from build123d import *

# Parameters (mm, degrees)
EXTRUDE_1931_DEPTH = 2


with BuildPart() as part:
    # Sketch 231 → Revolve 1 (revolve)
    with BuildSketch(Plane.XY, mode=Mode.PRIVATE) as revolve_1_sk:
        with BuildLine():
            Line((0, 11), (0, 0))
            Line((0, 0), (1, 0))
            Line((1, 0), (1, 5.25))
            Line((1, 5.25), (3.5, 5.25))
            Line((3.5, 5.25), (3.5, 0))
            Line((3.5, 0), (11.2, 0))
            Line((11.2, 0), (11.2, 4.8))
            ThreePointArc((11.2, 4.8), (10.2627417, 7.0627417), (8, 8))
            ThreePointArc((8, 8), (7.121320344, 10.121320344), (5, 11))
            Line((5, 11), (0, 11))
        make_face()
    revolve(revolve_1_sk.sketch.rotate(Axis((0, 0, 0), (1, 0, 0)), 90), axis=Axis((0, 0, 0), (1, 0, 0)))

    # Sketch 913 → Extrude 1931 (add, symmetric)
    with BuildSketch(Plane.XY):
        with BuildLine():
            ThreePointArc((11.2, 4.4), (29.338267199, 10.995701086), (45.2, 0))
            Line((45.2, 0), (11.2, 0))
            Line((11.2, 0), (11.2, 4.4))
        make_face()
        with BuildLine():
            Line((31.263463773, 0), (11.2, 0))
            Line((11.2, 0), (11.2, -3.914978255))
            ThreePointArc((11.2, -3.914978255), (22.080678837, -6.30816882), (31.263463773, 0))
        make_face()
        Polygon((38.912013935, 0), (35.248695767, 0), (35.248695767, -11.07), (38.912013935, -4.32), align=None)
        Polygon((35.248695767, 0), (31.263463773, 0), (32.498964702, -1.197255299), (32.498964702, -9.797255299), (35.248695767, -11.07), align=None)
        Polygon((42.083014277, -1.2), (42.083014277, 0), (40.307542508, 0), (40.307542508, -6.49), align=None)
        Polygon((40.307542508, 0), (38.912013935, 0), (38.912013935, -4.32), (40.307542508, -6.49), align=None)
        Polygon((42.083014277, -1.2), (45.2, 0), (42.083014277, 0), align=None)
    extrude(amount=EXTRUDE_1931_DEPTH, both=True)


solid = part.part
Build history of the part. All positions in model axes, mm. A direction names the side the tool comes from. Give positions to 0.01 mm unless a question says otherwise; leave off trailing zeros. Order: outer loops, then holes, each group sorted by start corner. A loop starts at its lowest first (then second) coordinate and runs counter-clockwise, first axis right, second up. Notation, with made-up numbers: M 83.25,51.25 L 90.25,51.25 A9 cw 90.25,65.25 Z; hole C -17,-15 d8. An arc over 180 degrees is marked long. Use one line per item in the form item = value.
Q1. Slice it at A-A, the plane y = -2.25. State how many separate pieces and enclosed holes the cut face has, and give its area (3 significant figures).
Conclusion:
separate_pieces = 2
enclosed_holes = 1
area = 299 mm2
Q2. Slice it at D-D, the plane x = 37. Write the cut outline in (y, z), and give its area (3 significant figures).
Conclusion:
outline = M -7.84,-2 L 8.44,-2 L 8.44,2 L -7.84,2 Z
area = 65.1 mm2
Q3. Pull direction Z, two halves, no side cores. Call faces 1 (the flat face through (28, 3, 2)), 2 (the flat face through (3.5, 0, 0)), 3 (the flat face through (1, 0, 0)), 4 (the flat face through (37.055, -7.742, 0.028)): released by +Z, released by -Z, zero draft, split by the parting line, or undercut.
Conclusion:
face_1 = released by +Z
face_2 = undercut
face_3 = undercut
face_4 = zero draft
Q4. Which spindle directions (+Z, -Z, +X, -X, +Y, -Y) get a long thin tool onto all of the face, cutting with end or side? Do faces 5 (the cylindrical face through (2.3, -1.6, 5)), 6 (the flat face through (39.6, -5.39, 0.03)), 7 (the flat face through (43.62, -0.61, 0.03)), 8 (the flat face through (0, 0, 0)), 9 (the flat face through (28, 3, -2)). Say none if no direction does.
Conclusion:
face_5 = none
face_6 = +Z, -Z, -Y
face_7 = +Z, -Z, +X, -Y
face_8 = +Z, -Z, -X, +Y, -Y
face_9 = -Z, +X, +Y, -Y
Q5. Wall check: probe 1 along Y at (x, z) = (2.85, 0); probe 2 along X at (y, z) = (-2, -2.5); probe 3 along Z at (x, y) = (42, 4). Give the ranges that are in metal, low to high.
Conclusion:
probe_1 = -11 to -5.25, 5.25 to 11
probe_2 = 0 to 1, 3.5 to 11.2
probe_3 = -2 to 2
Q6. Slice it at B-B, the plane z = 0. Write the cut outline in (x, y).
Conclusion:
outline = M 0,-11 L 5,-11 A3 ccw 8,-8 A3.2 ccw 11.2,-4.8 L 11.2,-3.91 A14 ccw 31.26,0 L 32.5,-1.2 L 32.5,-9.8 L 35.25,-11.07 L 38.91,-4.32 L 40.31,-6.49 L 42.08,-1.2 L 45.2,0 A21 ccw 11.2,4.4 L 11.2,4.8 A3.2 ccw 8,8 A3 ccw 5,11 L 0,11 Z; hole M 1,-5.25 L 3.5,-5.25 L 3.5,5.25 L 1,5.25 Z
Q7. Slice it at C-C, the plane x = 4. Write the cut outline in (y, z), and give its area (3 significant figures).
Conclusion:
outline = C 0,0 d22
area = 380 mm2
Q8. Pin check, flat tips, straight feed: P1, Ø2.5, axis at y = 0, z = 0, coming from the +X side; P2, Ø3, axis at y = -4.5, z = 2, coming from the +X side; P3, Ø5, axis at x = 11, z = 8, coming from the -Y side. Stop position of each tip, or through.
Conclusion:
P1 = 45.2
P2 = 41.48
P3 = -4.71
